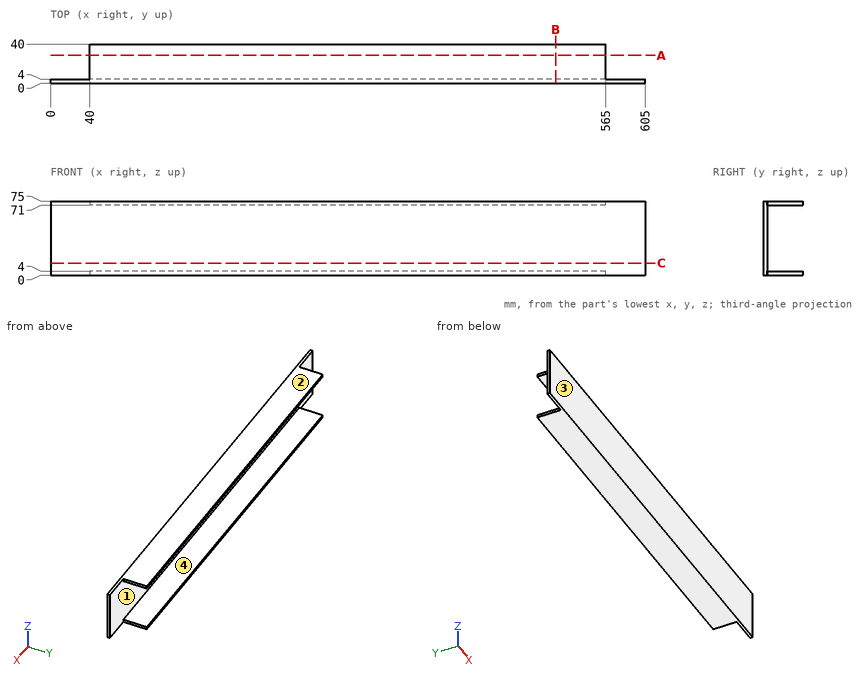
Geometry check sheet. Reference: drawing and pictorial views, mm from the part's lowest x, y, z. Give positions to 0.01 mm unless a question says otherwise; leave off trailing zeros. Order: outer loops, then holes, each group sorted by start corner. A loop starts at its lowest first (then second) coordinate and runs counter-clockwise, first axis right, second up. Notation, with made-up numbers: M -27.75,-16 L -8.75,-16 A22 cw -8.75,21 Z; hole C 79.5,84 d7. An arc over 180 degrees is marked long. Answer in a Markdown table with one row per item. Add a question column.
Q1. Gauge pin test, flat ends, axial feed: pin 1 Ø22.5 at (x, z) = (370, 37.5) entering from +Y; pin 2 Ø2 at (y, z) = (24, 73) entering from -X; pin 3 Ø3 at (y, z) = (27, 73.5) entering from +X. Record the tip position at first contact, or that the pin passes through.
Q2. Sectioned sample at C-C, the plane z = 12. Record the boundary of the cut face in (x, y), and give its area (3 significant figures).
Q3. Sectioned sample at A-A, the plane y = 28.5. Record the boundary of the cut face in (x, z).
Q4. Sectioned sample at B-B, the plane x = 514. Record the boundary of the cut face in (y, z).
Q5. Thickness scan on L1, parallel to Z at x = 266.5, y = 33.5; L2, parallel to Y at x = 323.5, z = 60. Record the ranges inside material, lowest first.
Q6. Release check for a two-part mould opening along Z. For the marked faces 1, 2, 3 and 4 record: released by +Z, released by -Z, zero draft, split by the parting line, or undercut.
Verdict:
| question | item | result |
|---|---|---|
| 1 | pin 1 | y = 4 |
| 1 | pin 2 | x = 40 |
| 1 | pin 3 | x = 565 |
| 2 | outline | M 0,0 L 605,0 L 605,4 L 0,4 Z |
| 2 | area | 2,420 mm² |
| 3 | outline | M 40,0 L 565,0 L 565,4 L 40,4 Z; M 40,71 L 565,71 L 565,75 L 40,75 Z |
| 4 | outline | M 0,0 L 40,0 L 40,4 L 4,4 L 4,71 L 40,71 L 40,75 L 0,75 Z |
| 5 | L1 | 0 to 4, 71 to 75 |
| 5 | L2 | 0 to 4 |
| 6 | face 1 | undercut |
| 6 | face 2 | released by +Z |
| 6 | face 3 | zero draft |
| 6 | face 4 | undercut |
